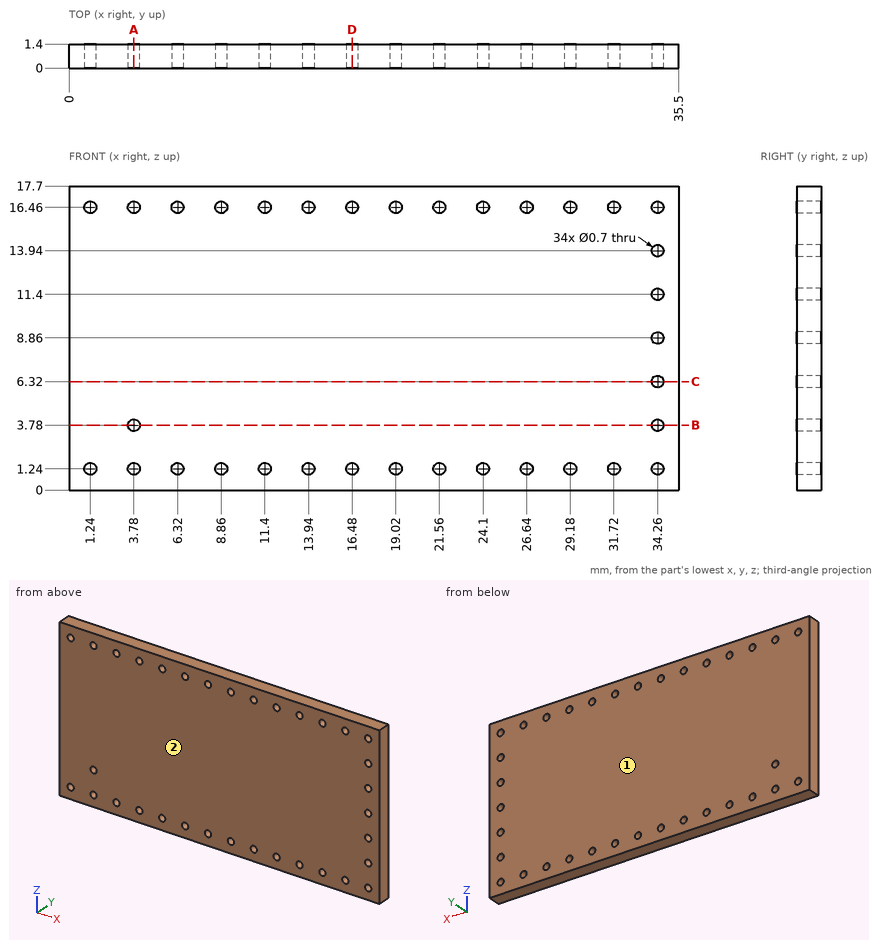
For this review, use the dimensioned drawing (mm, ordinates from the lowest corner) and the shaded views. Round coordinates to 2 decimals unless told otherwise and drop trailing zeros. Write each loop counter-clockwise with the first axis right and the second up, starting at its lowest first coordinate (ties: lowest second). Pieces come first, ordered by that corner, then holes. Notation, with made-up numbers: (-15, -33) - (-5, -33) arc R28 cw to (-5, 1) - close; hole circle Ø8 at (53.5, 64.5). An arc over 180 degrees is marked (long way). Use CSV: the item, a comma, the result in double quotes.
1) Add section C-C on z = 6.32. Write out the cut boundary in (x, y).
Conclusion:
outline,"(0, 0) - (33.91, 0) - (33.91, 1.4) - (0, 1.4) - close; (34.61, 0) - (35.5, 0) - (35.5, 1.4) - (34.61, 1.4) - close"
2) The part is to be moulded in two halves that separate along Y. For the marked faces 1 and 2, say which applies: pulls with the +Y half, pulls with the -Y half, needs draft (parallel to the pull), parting line crosses it, or undercut.
Conclusion:
face 1,"pulls with the +Y half"
face 2,"pulls with the -Y half"
3) Add section D-D on x = 16.48. Write out the cut boundary in (y, z).
Conclusion:
outline,"(0, 0) - (1.4, 0) - (1.4, 0.89) - (0, 0.89) - close; (0, 1.59) - (1.4, 1.59) - (1.4, 16.11) - (0, 16.11) - close; (0, 16.81) - (1.4, 16.81) - (1.4, 17.7) - (0, 17.7) - close"
4) Wall thickness on line 1 along X through (y, z) = (0.4, 3.78); line 2 along Z through (x, y) = (26.64, 0.85); line 3 along Z through (x, y) = (29, 0.75): over which ranges is each line inside the solid? List them lowest first. Write a range as from..to.
Conclusion:
line 1,"x = 0..3.43, 4.13..33.91, 34.61..35.5"
line 2,"z = 0..0.89, 1.59..16.11, 16.81..17.7"
line 3,"z = 0..0.94, 1.54..16.16, 16.76..17.7"
5) Add section A-A on x = 3.78. Write out the cut boundary in (y, z).
Conclusion:
outline,"(0, 0) - (1.4, 0) - (1.4, 0.89) - (0, 0.89) - close; (0, 1.59) - (1.4, 1.59) - (1.4, 3.43) - (0, 3.43) - close; (0, 4.13) - (1.4, 4.13) - (1.4, 16.11) - (0, 16.11) - close; (0, 16.81) - (1.4, 16.81) - (1.4, 17.7) - (0, 17.7) - close"
6) Add section B-B on z = 3.78. Write out the cut boundary in (x, y).
Conclusion:
outline,"(0, 0) - (3.43, 0) - (3.43, 1.4) - (0, 1.4) - close; (4.13, 0) - (33.91, 0) - (33.91, 1.4) - (4.13, 1.4) - close; (34.61, 0) - (35.5, 0) - (35.5, 1.4) - (34.61, 1.4) - close"
